Answer from the drawing. Dimensions are ordinates in mm from the lowest x, y and z of the part. A direction names the side the tool comes from. Coordinates: 2 decimals unless noted, no trailing zeros. Write each loop counter-clockwise with the first axis right and the second up, starting at its lowest first coordinate (ties: lowest second). Pieces come first, ordered by that corner, then holes. Notation, with made-up numbers: (86, 16.5) - (99, 16.5) arc R20 ccw to (99, 31.5) - close; hole circle Ø7 at (15, 47). An arc over 180 degrees is marked (long way). Use CSV: the item, a comma, the result in double quotes. Start each with the question number.
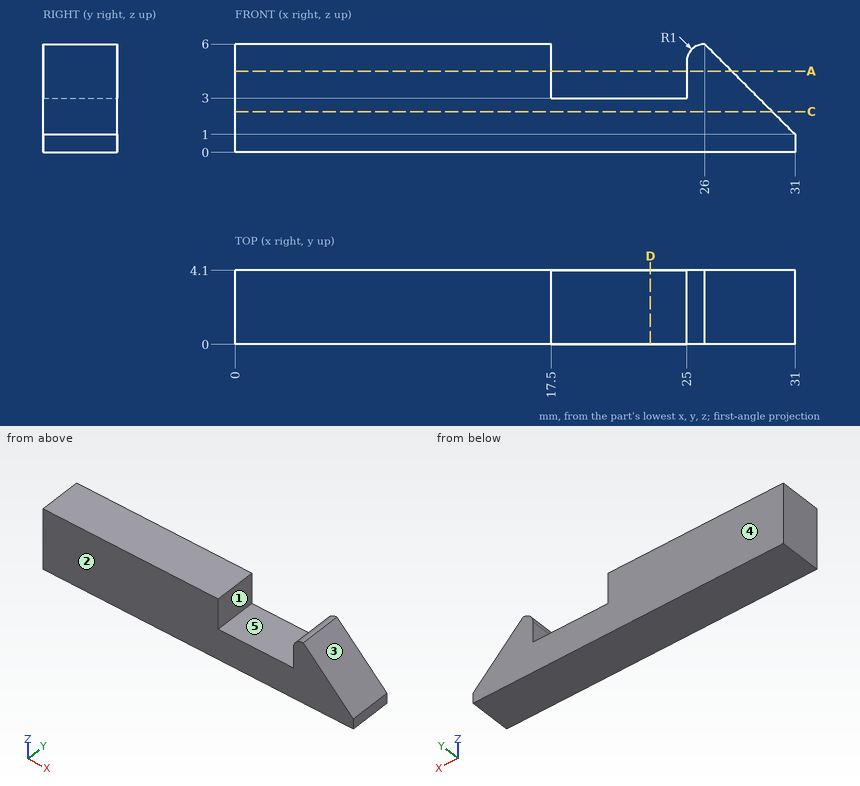
Item 1: A cutting plane is placed at C-C (z = 2.25). Determine the outline of the cut face in (x, y), then the cut area to 3 significant figures.
Item 2: Which of the six approach directions +Z, -Z, +X, -X, +Y, -Y give full straight-line access (tool end or side, diameter ignored) to the marked faces 1 and 2?
Item 3: Determine the mould class of the marked faces 3, 4 and 5 for opening direction X: +X half, -X half, draft (parallel to the pull), parting line (faces both ways), or undercut.
Item 4: A cutting plane is placed at A-A (z = 4.5). Determine the outline of the cut face in (x, y).
Item 5: A cutting plane is placed at D-D (x = 23). Determine the outline of the cut face in (y, z), then the cut area to 3 significant figures.
Item 6: Straight lines are drawn through the part: probe 1 along Z at (x, y) = (22.5, 3.8); probe 2 along Z at (x, y) = (27, 2.8); probe 3 along X at (y, z) = (3.75, 5.5) (1 decimal). For each, find the intervals that lie inside material, in ascending order. Write a range as [from, to].
Calculated:
1,outline,"(0, 0) - (29.75, 0) - (29.75, 4.1) - (0, 4.1) - close"
1,area,"122 mm²"
2,face 1,"+Z, +Y, -Y"
2,face 2,"+Z, -Z, +X, -X, -Y"
3,face 3,"+X half"
3,face 4,"draft"
3,face 5,"undercut"
4,outline,"(0, 0) - (17.5, 0) - (17.5, 4.1) - (0, 4.1) - close; (25, 0) - (27.5, 0) - (27.5, 4.1) - (25, 4.1) - close"
5,outline,"(0, 0) - (4.1, 0) - (4.1, 3) - (0, 3) - close"
5,area,"12.3 mm²"
6,probe 1,"z = [0, 3]"
6,probe 2,"z = [0, 5]"
6,probe 3,"x = [0, 17.5], [25.1, 26.5]"
